from build123d import *

# Parameters (mm, degrees)
F0_R     = 1.4
F0_R_2   = 3.925
F1_DEPTH = 2


with BuildPart() as f1:
    # F0 (on Front) → F1 (new body)
    with BuildSketch(Plane.XZ):
        with BuildLine():
            ThreePointArc((-3.882353, 6.10419), (-3.229356, 5.12965), (-3, 3.979203))
            Line((-3, 3.979203), (-3, 0))
            Line((-3, 0), (-3, -10))
            ThreePointArc((-3, -10), (0, -13), (3, -10))
            Line((3, -10), (3, 0))
            Line((3, 0), (3, 3.979203))
            ThreePointArc((3, 3.979203), (3.229356, 5.12965), (3.882353, 6.10419))
            ThreePointArc((3.882353, 6.10419), (0, 15.5), (-3.882353, 6.10419))
        make_face()
        with Locations((0, -10)):
            Circle(F0_R, mode=Mode.SUBTRACT)
        with Locations((0, 10)):
            Circle(F0_R_2, mode=Mode.SUBTRACT)
    extrude(amount=F1_DEPTH)


solid = f1.part
Verification items for the finished model (mm, model axes). A direction names the side the tool comes from. Coordinates: 2 decimals unless noted, no trailing zeros. Order: outer loops, then holes, each group sorted by start corner. A loop starts at its lowest first (then second) coordinate and runs counter-clockwise, first axis right, second up. Notation, with made-up numbers: (-11, 45.25) -> (3, 45.25) arc R9 ccw to (3, 62.25) -> close; hole circle Ø3 at (-29, 82.25). An arc over 180 degrees is marked (long way). Put each result on its own line as item: value. Start each with the question number.
1. Material ranges on L1, parallel to X at y = -0.9, z = -1.75; L2, parallel to Z at x = -2.75, y = -0.9; L3, parallel to Z at x = -3.5, y = -0.9, recorded low to high. Write a range as [from, to].
2. Cross-section at B-B, the plane z = 7.5. Record the boundary of the cut face in (x, y), then the cut area to 3 significant figures.
3. Cross-section at A-A, the plane x = 0. Record the boundary of the cut face in (y, z) (3 decimals), then the cut area to 3 significant figures.
4. Cross-section at D-D, the plane y = -1.05. Record the boundary of the cut face in (x, z) (3 decimals).
5. Cross-section at C-C, the plane x = 2.5. Record the boundary of the cut face in (y, z), then the cut area to 3 significant figures.
6. Mould release check, pull along X, two halves, no side actions. Record for faces 3 (the flat face through (0, -2, 1)), 4 (the flat face through (-3, -1, -3)), 5 (the cylindrical face through (-0.85, -0.99, 6.17)): released by +X, released by -X, zero draft, split by the parting line, or undercut.
7. Access from +Z, -Z, +X, -X, +Y, -Y to the whole of each face (thin tool, end or side, straight path). Record for faces 1 (the cylindrical face through (0.182, -0.986, 15.497)), 2 (the flat face through (3, -1, -3)).
8. Go/stop test with a flat-tipped pin: pin 1 Ø1 at (y, z) = (-1, 0) entering from +X. Record where the tip stops, or that it passes through.
Computed:
1. L1: [-3, 3]
1. L2: [-11.2, 7.2], [12.8, 14.76]
1. L3: [5.64, 8.22], [11.78, 14.24]
2. outline: (-4.9, -2) -> (-3.03, -2) -> (-3.03, 0) -> (-4.9, 0) -> close; (3.03, -2) -> (4.9, -2) -> (4.9, 0) -> (3.03, 0) -> close
2. area: 7.49 mm2
3. outline: (-2, -13) -> (0, -13) -> (0, -11.4) -> (-2, -11.4) -> close; (-2, -8.6) -> (0, -8.6) -> (0, 6.075) -> (-2, 6.075) -> close; (-2, 13.925) -> (0, 13.925) -> (0, 15.5) -> (-2, 15.5) -> close
3. area: 35.7 mm2
4. outline: (-3.882, 6.104) arc R3 cw to (-3, 3.979) -> (-3, -10) arc R3 ccw to (3, -10) -> (3, 3.979) arc R3 cw to (3.882, 6.104) arc R5.5 ccw (long way) to start; hole circle Ø7.85 at (0, 10); hole circle Ø2.8 at (0, -10)
5. outline: (-2, -11.66) -> (0, -11.66) -> (0, 6.97) -> (-2, 6.97) -> close; (-2, 13.03) -> (0, 13.03) -> (0, 14.9) -> (-2, 14.9) -> close
5. area: 41.0 mm2
6. face 3: zero draft
6. face 4: released by -X
6. face 5: undercut
7. face 1: +Y, -Y
7. face 2: -Z, +X, +Y, -Y
8. pin 1: x = 3
